For this review, take the finished solid that the model builds, in its own axes (mm). A direction names the side the tool comes from. Give positions to 0.01 mm unless a question says otherwise; leave off trailing zeros. Order: outer loops, then holes, each group sorted by start corner. A loop starts at its lowest first (then second) coordinate and runs counter-clockwise, first axis right, second up. Notation, with made-up numbers: M -23,-33.75 L 23,-33.75 A29 cw 23,-5.75 Z; hole C 22,-19.75 d7. An arc over 180 degrees is marked long. Use CSV: the item, a comma, the result in double quotes. Start each with the question number.
(1) Tool access review of faces 1 (the face through (315.95, 901.47, 27.76)), 2 (the face through (314, 900.56, 12)): name each direction out of +Z, -Z, +X, -X, +Y, -Y from which nothing blocks a thin tool from reaching the whole face with its end or side.
(2) Clearance check with flat-ended pins moving along their axes: P1, Ø5, axis at y = 880.5, z = 13.5, coming from the -X side; P2, Ø5, axis at x = 303, z = 23.5, coming from the -Y side; P3, Ø12, axis at x = 316.5, y = 889, coming from the +Z side; P4, Ø2, axis at x = 328, y = 902, coming from the +Z side. State where each tip first meets the part, or that it passes through.
(3) Consider section A-A (x = 322.5). Write out the cut boundary in (y, z), and give its area (3 significant figures).
(4) Consider section C-C (y = 899.5). Write out the cut boundary in (x, z).
(5) Consider section B-B (z = 23). Write out the cut boundary in (x, y).
(6) Wall thickness on L1, parallel to Y at x = 308.5, z = 9.5; L2, parallel to X at y = 896, z = 10.5; L3, parallel to Z at x = 321.5, y = 878: over which ranges is each line inside the solid? List them lowest first. Write a range as from..to.
(7) Consider section D-D (y = 904.5). Write out the cut boundary in (x, z), and give its area (3 significant figures).
```python
from build123d import *

# Parameters (mm, degrees)
REVOLVE1_ANGLE = 30


with BuildPart() as part:
    # Sketch1 → Revolve1 (revolve)
    with BuildSketch(Plane.XY):
        Polygon((297.869910117, 906.559895472), (332.869910117, 906.559895472), (332.869910117, 902.559895472), (332.869910117, 874.70937118), (326.869910117, 874.70937118), (326.869910117, 900.559895472), (297.869910117, 900.559895472), align=None)
    revolve(axis=Axis((267.869910117, 911.559895472, 0), (0, -1, 0)), revolution_arc=REVOLVE1_ANGLE)


solid = part.part
```
Check result:
1,face 1,"+Z, -X, +Y, -Y"
1,face 2,"-Z, -X, -Y"
2,P1,"stops at x = 324.66"
2,P2,"passes through"
2,P3,"stops at z = 31.54"
2,P4,"stops at z = 26.99"
3,outline,"M 874.71,22.28 L 900.56,22.28 L 900.56,0 L 906.56,0 L 906.56,31.54 L 874.71,31.54 Z"
3,area,"429 mm^2"
4,outline,"M 318.97,29.5 A59 cw 326.87,0 L 332.87,0 A65 ccw 324.16,32.5 Z"
5,outline,"M 307.71,900.56 L 322.2,900.56 L 322.2,874.71 L 328.66,874.71 L 328.66,906.56 L 307.71,906.56 Z"
6,L1,"y = 900.56..906.56"
6,L2,"x = 325.93..332.02"
6,L3,"z = 24.59..30.96"
7,outline,"M 293.85,15 A30 cw 297.87,0 L 332.87,0 A65 ccw 324.16,32.5 Z"
7,area,"870 mm^2"
